```python
from build123d import *

# Parameters (mm, degrees)
SKETCH018_W  = 5.4
SKETCH018_H  = 5.4
PAD012_DEPTH = 3
SKETCH020_W  = 6.1
SKETCH020_H  = 6.1
PAD013_DEPTH = 1.5
SKETCH021_R  = 1.1
PAD014_DEPTH = 2


with BuildPart() as part:
    # Sketch018 → Pad012 (new body)
    with BuildSketch(Plane.XY):
        with Locations((22.2, 0)):
            Rectangle(SKETCH018_W, SKETCH018_H)
    extrude(amount=PAD012_DEPTH)

    # Sketch020 → Pad013 (join)
    with BuildSketch(Plane.XY):
        with Locations((22.2, 0)):
            Rectangle(SKETCH020_W, SKETCH020_H)
    extrude(amount=-PAD013_DEPTH)

    # Sketch021 → Pad014 (join)
    with BuildSketch(Plane.XY):
        with Locations((22.2, 0)):
            Circle(SKETCH021_R)
    extrude(amount=-PAD014_DEPTH)


with BuildPart() as part_1:
    # Body006 placement: moved
    add(part.part.moved(Location((0, 32.5, 8.5))))


solid = part_1.part
```
Geometry check sheet. Reference: the model listing, model coordinates, mm. A direction names the side the tool comes from. Coordinates: 2 decimals unless noted, no trailing zeros. Write each loop counter-clockwise with the first axis right and the second up, starting at its lowest first coordinate (ties: lowest second). Pieces come first, ordered by that corner, then holes. Notation, with made-up numbers: M 5.25,-38.75 L 36.25,-38.75 A19 ccw 36.25,-23.75 Z; hole C -7.75,70 d8. An arc over 180 degrees is marked long. One line per item, written item: value. Start each with the question number.
(1) Sectioned sample at B-B, the plane x = 22.2. Enter the section's corners in (y, z), and give its area (4 significant figures).
(2) Tool access check on faces 1 (the face through (24.9, 32, 10)), 2 (the face through (22, 35.2, 10)), 3 (the face through (22.79, 33.43, 6.75)), 4 (the face through (22, 29.8, 10)), 5 (the face through (19.5, 32, 10)). Record the directions out of +Z, -Z, +X, -X, +Y, -Y that give a thin tool (end or side, any length) a straight path to the whole face; none if there is none.
(3) Sectioned sample at A-A, the plane y = 31.25. Enter the section's corners in (x, z).
(4) Scan lines: line 1 along Y through (x, z) = (21, 8.65); line 2 along Z through (x, y) = (21.5, 31.5); line 3 along X through (y, z) = (31.25, 10.55). Record each from-to range of solid material in increasing order. Write a range as [from, to].
(5) Sectioned sample at C-C, the plane z = 10.4. Enter the section's corners in (x, y), and give its area (3 significant figures).
(6) Sectioned sample at D-D, the plane x = 24.5. Enter the section's corners in (y, z), and give its area (4 significant figures).
(7) Depth check by flat-ended pin: pin 1 (1 mm diameter, centred on x = 20, y = 32, fed in from -Z); pin 2 (1.5 mm diameter, centred on x = 21.5, z = 10, fed in from +Y); pin 3 (0.9 mm diameter, centred on x = 21.5, z = 10, fed in from -Y). Enter the tip coordinate at first touch or a pass-through.
Filled sheet:
1. outline: M 29.45,7 L 31.4,7 L 31.4,6.5 L 33.6,6.5 L 33.6,7 L 35.55,7 L 35.55,8.5 L 35.2,8.5 L 35.2,11.5 L 29.8,11.5 L 29.8,8.5 L 29.45,8.5 Z
1. area: 26.45 mm²
2. face 1: +Z, +X, +Y, -Y
2. face 2: +Z, +X, -X, +Y
2. face 3: -Z
2. face 4: +Z, +X, -X, -Y
2. face 5: +Z, -X, +Y, -Y
3. outline: M 19.15,7 L 25.25,7 L 25.25,8.5 L 24.9,8.5 L 24.9,11.5 L 19.5,11.5 L 19.5,8.5 L 19.15,8.5 Z
4. line 1: [29.8, 35.2]
4. line 2: [7, 11.5]
4. line 3: [19.5, 24.9]
5. outline: M 19.5,29.8 L 24.9,29.8 L 24.9,35.2 L 19.5,35.2 Z
5. area: 29.2 mm²
6. outline: M 29.45,7 L 35.55,7 L 35.55,8.5 L 35.2,8.5 L 35.2,11.5 L 29.8,11.5 L 29.8,8.5 L 29.45,8.5 Z
6. area: 25.35 mm²
7. pin 1: z = 7
7. pin 2: y = 35.2
7. pin 3: y = 29.8
